from build123d import *

# Parameters (mm, degrees)
F0_R     = 101.6
F0_R_2   = 6.35
F1_DEPTH = 25.4


with BuildPart() as f1:
    # F0 (on Front) → F1 (new body)
    with BuildSketch(Plane.XZ):
        Circle(F0_R)
        with Locations((-38.790503, -65.587628)):
            Circle(F0_R_2, mode=Mode.SUBTRACT)
        Polygon((16.131167, 0), (8.065583, -13.97), (-8.065583, -13.97), (-16.131167, 0), (-8.065583, 13.97), (8.065583, 13.97), align=None, mode=Mode.SUBTRACT)
        with Locations((37.4053, -66.387375)):
            Circle(F0_R_2, mode=Mode.SUBTRACT)
        with Locations((76.195803, -0.799747)):
            Circle(F0_R_2, mode=Mode.SUBTRACT)
        with Locations((-76.195803, 0.799747)):
            Circle(F0_R_2, mode=Mode.SUBTRACT)
        with Locations((-37.4053, 66.387375)):
            Circle(F0_R_2, mode=Mode.SUBTRACT)
        with Locations((38.790503, 65.587628)):
            Circle(F0_R_2, mode=Mode.SUBTRACT)
    extrude(amount=F1_DEPTH)


solid = f1.part
Work out the finished part from the listing and answer in its coordinate system (mm). A direction names the side the tool comes from. Give positions to 0.01 mm unless a question says otherwise; leave off trailing zeros. Loops run counter-clockwise (first coordinate to the right, second up) from the corner with the lowest first, then second, coordinate; pieces in that order, holes last. Notation, with made-up numbers: (82.25, -11.75) -> (140.25, -11.75) arc R16 cw to (140.25, 1.25) -> close; hole circle Ø2 at (-7.75, -26). An arc over 180 degrees is marked (long way). Use a Markdown table: item, result. Add a question column.
1) The part is cut by section B-B, the plane x = 35.5. Determine the outline of the cut face in (y, z), plus the area to 3 significant figures.
2) Each of these flat-tipped pins is pushed along its axis until it touches: P1, Ø3, axis at y = -9, z = 49, coming from the -X side; P2, Ø4, axis at x = 58, y = -7, coming from the -Z side; P3, Ø4, axis at y = -21, z = 15, coming from the +X side; P4, Ø10, axis at x = 38.79, z = 65.59, coming from the +Y side. Where does it stop, or does it pass through?
3) The part is cut by section A-A, the plane x = 0. Determine the outline of the cut face in (y, z).
4) Consider line 1 along X through (y, z) = (-23.5, 64); line 2 along Z through (x, y) = (-2, -23); line 3 along Z through (x, y) = (-36.5, -18.5). Determine where each line is inside the solid, lowest interval first.
5) Which of the six approach directions +Z, -Z, +X, -X, +Y, -Y give full straight-line access (tool end or side, diameter ignored) to faces 5 (the flat face through (-1, 0, -21)), 6 (the flat face through (0, -13, 13.97))?
6) The part is cut by section D-D, the plane z = -41. Determine the outline of the cut face in (x, y), plus the area to 3 significant figures.
7) The part is cut by section C-C, the plane y = -20.5. Determine the outline of the cut face in (x, z).
8) For a pull along X with two mould halves and no side action, classify faces 1 (the cylindrical face through (-70.14, -12.52, 2.71)), 2 (the cylindrical face through (-22.025, -12.522, -99.184)), 3 (the flat face through (-1, -25.4, -21)), 4 (the flat face through (-12.155, -12.522, 6.887)) as +X half, -X half, draft (parallel to the pull), parting line (faces both ways), or undercut.
Reported:
| question | item | result |
|---|---|---|
| 1 | outline | (-25.4, -95.2) -> (0, -95.2) -> (0, -72.44) -> (-25.4, -72.44) -> close; (-25.4, -60.33) -> (0, -60.33) -> (0, 60.16) -> (-25.4, 60.16) -> close; (-25.4, 71.02) -> (0, 71.02) -> (0, 95.2) -> (-25.4, 95.2) -> close |
| 1 | area | 4,250 mm^2 |
| 2 | P1 | stops at x = -89.81 |
| 2 | P2 | stops at z = -84.77 |
| 2 | P3 | stops at x = 100.76 |
| 2 | P4 | passes through |
| 3 | outline | (-25.4, -101.6) -> (0, -101.6) -> (0, -13.97) -> (-25.4, -13.97) -> close; (-25.4, 13.97) -> (0, 13.97) -> (0, 101.6) -> (-25.4, 101.6) -> close |
| 4 | line 1 | x = -78.91 to -43.29, -31.52 to 32.64, 44.94 to 78.91 |
| 4 | line 2 | z = -101.58 to -13.97, 13.97 to 101.58 |
| 4 | line 3 | z = -94.82 to -71.51, -59.67 to 60.1, 72.67 to 94.82 |
| 5 | face 5 | +Z, -Z, +X, -X, +Y |
| 5 | face 6 | +Y, -Y |
| 6 | outline | (-92.96, -25.4) -> (92.96, -25.4) -> (92.96, 0) -> (-92.96, 0) -> close |
| 6 | area | 4,720 mm^2 |
| 7 | outline | circle Ø203.2 at (0, 0); hole circle Ø12.7 at (-76.2, 0.8); hole circle Ø12.7 at (-38.79, -65.59); hole circle Ø12.7 at (-37.41, 66.39); hole (-16.13, 0) -> (-8.07, -13.97) -> (8.07, -13.97) -> (16.13, 0) -> (8.07, 13.97) -> (-8.07, 13.97) -> close; hole circle Ø12.7 at (37.41, -66.39); hole circle Ø12.7 at (38.79, 65.59); hole circle Ø12.7 at (76.2, -0.8) |
| 8 | face 1 | undercut |
| 8 | face 2 | parting line |
| 8 | face 3 | draft |
| 8 | face 4 | undercut |
